Work out the finished part from the listing and answer in its coordinate system (mm). A direction names the side the tool comes from. Give positions to 0.01 mm unless a question says otherwise; leave off trailing zeros. Order: outer loops, then holes, each group sorted by start corner. A loop starts at its lowest first (then second) coordinate and runs counter-clockwise, first axis right, second up.
```python
from build123d import *

# Parameters (mm, degrees)
SKETCH_1_R      = 1.5
EXTRUDE_1_DEPTH = 2


with BuildPart() as part:
    # 草图1 → 凸台-拉伸1 (new body)
    with BuildSketch(Plane(origin=(0, 0, 0), x_dir=(1, 0, 0), z_dir=(0, 1, 0))):
        with BuildLine():
            Line((-49.990380792, -29.946956811), (49.990380792, -29.946956811))
            ThreePointArc((49.990380792, -29.946956811), (54.239823286, -28.186780098), (56, -23.937337603))
            Line((56, -23.937337603), (56, 24.043423981))
            ThreePointArc((56, 24.043423981), (54.239823286, 28.292866475), (49.990380792, 30.053043189))
            Line((49.990380792, 30.053043189), (34.49744459, 30.053043189))
            ThreePointArc((34.49744459, 30.053043189), (33.085037975, 30.638081164), (32.5, 32.050487778))
            Line((32.5, 32.050487778), (32.5, 36.050487778))
            ThreePointArc((32.5, 36.050487778), (31.914213562, 37.464701341), (30.5, 38.050487778))
            Line((30.5, 38.050487778), (-30.5, 38.050487778))
            ThreePointArc((-30.5, 38.050487778), (-31.914213562, 37.464701341), (-32.5, 36.050487778))
            Line((-32.5, 36.050487778), (-32.5, 32.050487778))
            ThreePointArc((-32.5, 32.050487778), (-33.085037975, 30.638081164), (-34.49744459, 30.053043189))
            Line((-34.49744459, 30.053043189), (-49.990380792, 30.053043189))
            ThreePointArc((-49.990380792, 30.053043189), (-54.239823286, 28.292866475), (-56, 24.043423981))
            Line((-56, 24.043423981), (-56, -23.937337603))
            ThreePointArc((-56, -23.937337603), (-54.239823286, -28.186780098), (-49.990380792, -29.946956811))
        make_face()
        with Locations(Location((27.37, 33.395487778, 0), (0, 0, 270))):
            Circle(SKETCH_1_R, mode=Mode.SUBTRACT)
        with Locations(Location((27.37, -10.294512222, 0), (0, 0, 270))):
            Circle(SKETCH_1_R, mode=Mode.SUBTRACT)
        with Locations(Location((53, 13.050487778, 0), (0, 0, 270))):
            Circle(SKETCH_1_R, mode=Mode.SUBTRACT)
        with Locations(Location((53, -12.949512222, 0), (0, 0, 270))):
            Circle(SKETCH_1_R, mode=Mode.SUBTRACT)
        with Locations(Location((35.500000351, -25.346956811, 0), (0, 0, 270))):
            Circle(SKETCH_1_R, mode=Mode.SUBTRACT)
        with Locations(Location((-27.37, 33.395487778, 0), (0, 0, 270))):
            Circle(SKETCH_1_R, mode=Mode.SUBTRACT)
        with Locations(Location((-53, 9.050487778, 0), (0, 0, 270))):
            Circle(SKETCH_1_R, mode=Mode.SUBTRACT)
        with Locations(Location((-53, -8.949512222, 0), (0, 0, 270))):
            Circle(SKETCH_1_R, mode=Mode.SUBTRACT)
        with Locations(Location((-35.499999649, -25.346956811, 0), (0, 0, 270))):
            Circle(SKETCH_1_R, mode=Mode.SUBTRACT)
        with Locations(Location((-27.37, -10.294512222, 0), (0, 0, 270))):
            Circle(SKETCH_1_R, mode=Mode.SUBTRACT)
        with Locations(Location((-44.07, -25.346956811, 0), (0, 0, 270))):
            Circle(SKETCH_1_R, mode=Mode.SUBTRACT)
        with Locations(Location((44.07, -25.346956811, 0), (0, 0, 270))):
            Circle(SKETCH_1_R, mode=Mode.SUBTRACT)
        with Locations(Location((-44.07, 25.453043189, 0), (0, 0, 270))):
            Circle(SKETCH_1_R, mode=Mode.SUBTRACT)
        with Locations(Location((-47.57, 25.453043189, 0), (0, 0, 270))):
            Circle(SKETCH_1_R, mode=Mode.SUBTRACT)
        with Locations(Location((-40.57, 25.453043189, 0), (0, 0, 270))):
            Circle(SKETCH_1_R, mode=Mode.SUBTRACT)
        with Locations(Location((44.07, 25.453043189, 0), (0, 0, 270))):
            Circle(SKETCH_1_R, mode=Mode.SUBTRACT)
        with Locations(Location((47.57, 25.453043189, 0), (0, 0, 270))):
            Circle(SKETCH_1_R, mode=Mode.SUBTRACT)
        with Locations(Location((40.57, 25.453043189, 0), (0, 0, 270))):
            Circle(SKETCH_1_R, mode=Mode.SUBTRACT)
        with BuildLine():
            Line((-46, -19.949512222), (-18.5, -19.949512222))
            ThreePointArc((-18.5, -19.949512222), (-17.085786438, -19.363725784), (-16.5, -17.949512222))
            Line((-16.5, -17.949512222), (-16.5, -16.949512222))
            ThreePointArc((-16.5, -16.949512222), (-17.085786438, -15.535298659), (-18.5, -14.949512222))
            Line((-18.5, -14.949512222), (-30.5, -14.949512222))
            ThreePointArc((-30.5, -14.949512222), (-31.914213562, -14.363725784), (-32.5, -12.949512222))
            Line((-32.5, -12.949512222), (-32.5, 20.08975605))
            Line((-32.5, 20.08975605), (-46, 20.08975605))
            ThreePointArc((-46, 20.08975605), (-48.121320344, 19.211076394), (-49, 17.08975605))
            Line((-49, 17.08975605), (-49, -16.949512222))
            ThreePointArc((-49, -16.949512222), (-48.121320344, -19.070832565), (-46, -19.949512222))
        make_face(mode=Mode.SUBTRACT)
        with BuildLine():
            Line((49, -16.949512222), (49, 17.08975605))
            ThreePointArc((49, 17.08975605), (48.121320344, 19.211076394), (46, 20.08975605))
            Line((46, 20.08975605), (32.5, 20.08975605))
            Line((32.5, 20.08975605), (32.5, -12.949512222))
            ThreePointArc((32.5, -12.949512222), (31.914213562, -14.363725784), (30.5, -14.949512222))
            Line((30.5, -14.949512222), (18.5, -14.949512222))
            ThreePointArc((18.5, -14.949512222), (17.085786438, -15.535298659), (16.5, -16.949512222))
            Line((16.5, -16.949512222), (16.5, -17.949512222))
            ThreePointArc((16.5, -17.949512222), (17.085786438, -19.363725784), (18.5, -19.949512222))
            Line((18.5, -19.949512222), (46, -19.949512222))
            ThreePointArc((46, -19.949512222), (48.121320344, -19.070832565), (49, -16.949512222))
        make_face(mode=Mode.SUBTRACT)
        with BuildLine():
            Line((-17, 30.300487778), (17, 30.300487778))
            ThreePointArc((17, 30.300487778), (19.121320344, 29.421808122), (20, 27.300487778))
            Line((20, 27.300487778), (20, -1.699512222))
            ThreePointArc((20, -1.699512222), (19.121320344, -3.820832565), (17, -4.699512222))
            Line((17, -4.699512222), (-17, -4.699512222))
            ThreePointArc((-17, -4.699512222), (-19.121320344, -3.820832565), (-20, -1.699512222))
            Line((-20, -1.699512222), (-20, 27.300487778))
            ThreePointArc((-20, 27.300487778), (-19.121320344, 29.421808122), (-17, 30.300487778))
        make_face(mode=Mode.SUBTRACT)
        with BuildLine():
            Line((47.5, -23.846956811), (49.5, -23.846956811))
            ThreePointArc((49.5, -23.846956811), (51, -25.346956811), (49.5, -26.846956811))
            Line((49.5, -26.846956811), (47.5, -26.846956811))
            ThreePointArc((47.5, -26.846956811), (46, -25.346956811), (47.5, -23.846956811))
        make_face(mode=Mode.SUBTRACT)
        with BuildLine():
            Line((-47.5, -23.839893014), (-49.5, -23.839893014))
            ThreePointArc((-49.5, -23.839893014), (-51.007063798, -25.346956811), (-49.5, -26.854020609))
            Line((-49.5, -26.854020609), (-47.5, -26.854020609))
            ThreePointArc((-47.5, -26.854020609), (-45.992936202, -25.346956811), (-47.5, -23.839893014))
        make_face(mode=Mode.SUBTRACT)
    extrude(amount=EXTRUDE_1_DEPTH)


solid = part.part
```
1. The part is cut by section C-C (z = 3). Write down the section's boundary in (x, y).
Findings below:
outline: (-56, 0) - (-49, 0) - (-49, 2) - (-56, 2) - close; (-32.5, 0) - (-19.7, 0) - (-19.7, 2) - (-32.5, 2) - close; (19.7, 0) - (32.5, 0) - (32.5, 2) - (19.7, 2) - close; (49, 0) - (56, 0) - (56, 2) - (49, 2) - close
2. The part is cut by section A-A (x = -40.57). Write down the section's boundary in (y, z), then the cut area to 3 significant figures.
Findings below:
outline: (0, -30.05) - (2, -30.05) - (2, -26.95) - (0, -26.95) - close; (0, -23.95) - (2, -23.95) - (2, -20.09) - (0, -20.09) - close; (0, 19.95) - (2, 19.95) - (2, 29.95) - (0, 29.95) - close
area: 33.9 mm2
3. Straight lines are drawn through the part: probe 1 along X at (y, z) = (0.55, -4.5); probe 2 along X at (y, z) = (0.6, 5.5); probe 3 along Z at (x, y) = (11.5, 1.55). For each, find the intervals that lie inside material, in ascending order.
Findings below:
probe 1: x = -56 to -49, -32.5 to -20, 20 to 32.5, 49 to 56
probe 2: x = -56 to -49, -32.5 to 32.5, 49 to 56
probe 3: z = -38.05 to -30.3, 4.7 to 29.95
4. The mould has two halves that part along X. Classify faces 1 (the face through (-34.013, 0.986, 25.152)), 2 (the face through (-32.5, 1, -34)), 3 (the face through (17.1, 0.99, 15.52)), 4 (the face through (56, 1, 0)): pulls with the +X half, pulls with the -X half, needs draft (parallel to the pull), parting line crosses it, or undercut.
Findings below:
face 1: undercut
face 2: pulls with the -X half
face 3: undercut
face 4: pulls with the +X half
5. The part is cut by section B-B (x = -5). Write down the section's boundary in (y, z).
Findings below:
outline: (0, -38.05) - (2, -38.05) - (2, -30.3) - (0, -30.3) - close; (0, 4.7) - (2, 4.7) - (2, 29.95) - (0, 29.95) - close
6. Given P1, Ø1, axis at x = 43.5, y = 1, coming from the -Z side, flat-ended and moving along its own axis, determine where the tip first touches the part or whether it passes through.
Findings below:
P1: stops at z = -30.05
7. Which of the six approach directions +Z, -Z, +X, -X, +Y, -Y give full straight-line access (tool end or side, diameter ignored) to faces 5 (the face through (31.93, 0.99, -37.45)), 6 (the face through (46, 1, 25.4))?
Findings below:
face 5: -Z, +X, +Y, -Y
face 6: +Y, -Y
8. The part is cut by section D-D (x = 27.37). Write down the section's boundary in (y, z).
Findings below:
outline: (0, -38.05) - (2, -38.05) - (2, -34.9) - (0, -34.9) - close; (0, -31.9) - (2, -31.9) - (2, 8.79) - (0, 8.79) - close; (0, 11.79) - (2, 11.79) - (2, 14.95) - (0, 14.95) - close; (0, 19.95) - (2, 19.95) - (2, 29.95) - (0, 29.95) - close
